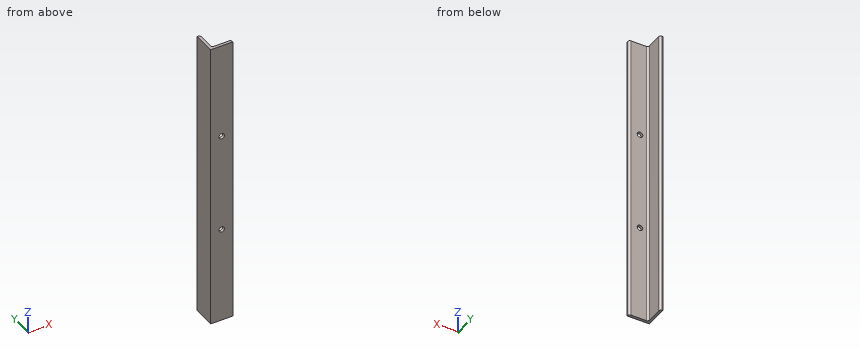
from build123d import *

# Parameters (mm, degrees)
BOSS_EXTRUDE1_DEPTH = 336.55
SKETCH2_R           = 6.35
CUT_EXTRUDE1_DEPTH  = 51.8


with BuildPart() as part:
    # Sketch1 → Boss-Extrude1 (new body, symmetric)
    with BuildSketch(Plane.XY):
        with BuildLine():
            Line((0, 0), (0, 50.8))
            Line((0, 50.8), (1.59258, 50.8))
            ThreePointArc((1.59258, 50.8), (4.956583943, 49.406583943), (6.35, 46.04258))
            Line((6.35, 46.04258), (6.35, 11.1125))
            ThreePointArc((6.35, 11.1125), (7.744903955, 7.744903955), (11.1125, 6.35))
            Line((11.1125, 6.35), (46.04258, 6.35))
            ThreePointArc((46.04258, 6.35), (49.406583943, 4.956583943), (50.8, 1.59258))
            Line((50.8, 1.59258), (50.8, 0))
            Line((50.8, 0), (0, 0))
        make_face()
    extrude(amount=BOSS_EXTRUDE1_DEPTH, both=True)

    # Sketch2 → Cut-Extrude1 (cut, through all)
    with BuildSketch(Plane.XZ):
        with Locations((25.4, -114.3)):
            Circle(SKETCH2_R)
        with Locations((25.4, 114.3)):
            Circle(SKETCH2_R)
    extrude(amount=-CUT_EXTRUDE1_DEPTH, mode=Mode.SUBTRACT)


solid = part.part
For this review, take the finished solid that the model builds, in its own axes (mm). Round coordinates to 2 decimals unless told otherwise and drop trailing zeros. Write each loop counter-clockwise with the first axis right and the second up, starting at its lowest first coordinate (ties: lowest second). Pieces come first, ordered by that corner, then holes. Notation, with made-up numbers: M 38.25,48.5 L 96.25,48.5 A25 cw 96.25,71.5 Z; hole C -38,86 d4. An arc over 180 degrees is marked long. Write item = value, one per line. Start each with the question number.
(1) For line 1 along Z through (x, y) = (25, 2); line 2 along X through (y, z) = (2, 114); line 3 along Y through (x, z) = (20.5, 105), list the stretches that pass through material, from the lowest coordinate up.
(2) We need section D-D (y = 19). Give the boundary of the cut face in (x, z).
(3) We need section B-B (x = 25.4). Give the boundary of the cut face in (y, z).
(4) Clearance check with flat-ended pins moving along their axes: pin 1 Ø10.5 at (x, z) = (30.5, 97.5) entering from +Y; pin 2 Ø10 at (x, z) = (25.4, -114.3) entering from -Y (3 decimals); pin 3 Ø5 at (y, z) = (37.5, -128.5) entering from +X; pin 4 Ø12 at (y, z) = (11, -72) entering from +X. State where each tip first meets the part, or that it passes through.
Results found:
q1.line_1 = -336.55 to -120.64, -107.96 to 107.96, 120.64 to 336.55
q1.line_2 = 0 to 19.06, 31.74 to 50.78
q1.line_3 = 0 to 6.35
q2.outline = M 0,-336.55 L 6.35,-336.55 L 6.35,336.55 L 0,336.55 Z
q3.outline = M 0,-336.55 L 6.35,-336.55 L 6.35,-120.65 L 0,-120.65 Z; M 0,-107.95 L 6.35,-107.95 L 6.35,107.95 L 0,107.95 Z; M 0,120.65 L 6.35,120.65 L 6.35,336.55 L 0,336.55 Z
q4.pin_1 = 6.35
q4.pin_2 = through
q4.pin_3 = 6.35
q4.pin_4 = 49.36
